Read the model definition and answer for the solid it produces. Units are mm, in the model's axes. A direction names the side the tool comes from. Give positions to 0.01 mm unless a question says otherwise; leave off trailing zeros. Use a Markdown table: item, result. Add a question column.
1. A cutting plane is placed at A-A on z = 4. State how many separate pieces and enclosed holes the cut face has, and give its area (3 significant figures).
2. Consider L1, parallel to X at y = 28.5, z = 4.75; L2, parallel to Z at x = 20.5, y = 29. Determine where each line is inside the solid, lowest interval first.
3. Flat-ended cylindrical pins translate along their axes: P1, Ø1, axis at x = 7, z = 4.5, coming from the -Y side; P2, Ø0.8, axis at x = 43, y = 6.5, coming from the +Z side; P3, Ø2.5, axis at x = 26.5, y = 75, coming from the +Z side. Find the tip coordinate at first contact, or state that the pin passes through.
4. For a pull along Y with two mould halves and no side action, classify faces 1 (the flat face through (24, 79, 6.35)), 2 (the flat face through (24, 81.28, 3)), 3 (the flat face through (25, 61.976, 5)), 4 (the flat face through (9, 37, 5.08)) as released by +Y, released by -Y, zero draft, split by the parting line, or undercut.
5. Which of the six approach directions +Z, -Z, +X, -X, +Y, -Y give full straight-line access (tool end or side, diameter ignored) to faces 5 (the flat face through (18.669, 36.8, 4.7)), 6 (the flat face through (24, 33, 6.35))?
```python
from build123d import *

# Parameters (mm, degrees)
F0_W     = 49.53
F0_H     = 81.28
F1_DEPTH = 6.35
F2_W     = 12.192
F2_H     = 4.572
F3_DEPTH = 3.302
F4_W     = 18.669
F4_H     = 1.524
F5_DEPTH = 1.27


with BuildPart() as f1:
    # F0 (on Top) → F1 (new body)
    with BuildSketch(Plane.XY):
        with Locations((24.765, 40.64)):
            Rectangle(F0_W, F0_H)
    extrude(amount=F1_DEPTH)

    # F2 (on face) → F3 (cut)
    with BuildSketch(Plane.XY.offset(6.35)):
        with Locations((24.765, 6.35)):
            Rectangle(F2_W, F2_H)
        with Locations((24.765, 13.97)):
            Rectangle(F2_W, F2_H)
        with Locations((24.765, 21.59)):
            Rectangle(F2_W, F2_H)
        with Locations((24.765, 29.21)):
            Rectangle(F2_W, F2_H)
        with Locations((24.765, 36.83)):
            Rectangle(F2_W, F2_H)
        with Locations((24.765, 44.45)):
            Rectangle(F2_W, F2_H)
        with Locations((24.765, 52.07)):
            Rectangle(F2_W, F2_H)
        with Locations((24.765, 59.69)):
            Rectangle(F2_W, F2_H)
        with Locations((24.765, 67.31)):
            Rectangle(F2_W, F2_H)
        with Locations((24.765, 74.93)):
            Rectangle(F2_W, F2_H)
    extrude(amount=-F3_DEPTH, mode=Mode.SUBTRACT)

    # F4 (on face) → F5 (cut)
    with BuildSketch(Plane.XY.offset(6.35)):
        with Locations((40.1955, 6.35)):
            Rectangle(F4_W, F4_H)
        with Locations((9.3345, 6.35)):
            Rectangle(F4_W, F4_H)
        with Locations((9.3345, 13.97)):
            Rectangle(F4_W, F4_H)
        with Locations((40.1955, 13.97)):
            Rectangle(F4_W, F4_H)
        with Locations((9.3345, 21.59)):
            Rectangle(F4_W, F4_H)
        with Locations((40.1955, 21.59)):
            Rectangle(F4_W, F4_H)
        with Locations((9.3345, 29.21)):
            Rectangle(F4_W, F4_H)
        with Locations((40.1955, 29.21)):
            Rectangle(F4_W, F4_H)
        with Locations((9.3345, 36.83)):
            Rectangle(F4_W, F4_H)
        with Locations((40.1955, 36.83)):
            Rectangle(F4_W, F4_H)
        with Locations((9.3345, 44.45)):
            Rectangle(F4_W, F4_H)
        with Locations((40.1955, 44.45)):
            Rectangle(F4_W, F4_H)
        with Locations((9.3345, 52.07)):
            Rectangle(F4_W, F4_H)
        with Locations((40.1955, 52.07)):
            Rectangle(F4_W, F4_H)
        with Locations((9.3345, 59.69)):
            Rectangle(F4_W, F4_H)
        with Locations((40.1955, 59.69)):
            Rectangle(F4_W, F4_H)
        with Locations((9.3345, 67.31)):
            Rectangle(F4_W, F4_H)
        with Locations((40.1955, 67.31)):
            Rectangle(F4_W, F4_H)
        with Locations((9.3345, 74.93)):
            Rectangle(F4_W, F4_H)
        with Locations((40.1955, 74.93)):
            Rectangle(F4_W, F4_H)
    extrude(amount=-F5_DEPTH, mode=Mode.SUBTRACT)


solid = f1.part
```
Output values:
| question | item | result |
|---|---|---|
| 1 | separate pieces | 1 |
| 1 | enclosed holes | 10 |
| 1 | area | 3,470 mm² |
| 2 | L1 | 0 to 18.67, 30.86 to 49.53 |
| 2 | L2 | 0 to 3.05 |
| 3 | P1 | y = 0 |
| 3 | P2 | z = 5.08 |
| 3 | P3 | z = 3.05 |
| 4 | face 1 | zero draft |
| 4 | face 2 | released by +Y |
| 4 | face 3 | undercut |
| 4 | face 4 | undercut |
| 5 | face 5 | +Z |
| 5 | face 6 | +Z, +X, -X, +Y, -Y |
